Study the drawing (mm; zero at the part's minimum x, y, z) and answer. Round coordinates to 2 decimals unless told otherwise and drop trailing zeros. Write each loop counter-clockwise with the first axis right and the second up, starting at its lowest first coordinate (ties: lowest second). Pieces come first, ordered by that corner, then holes.
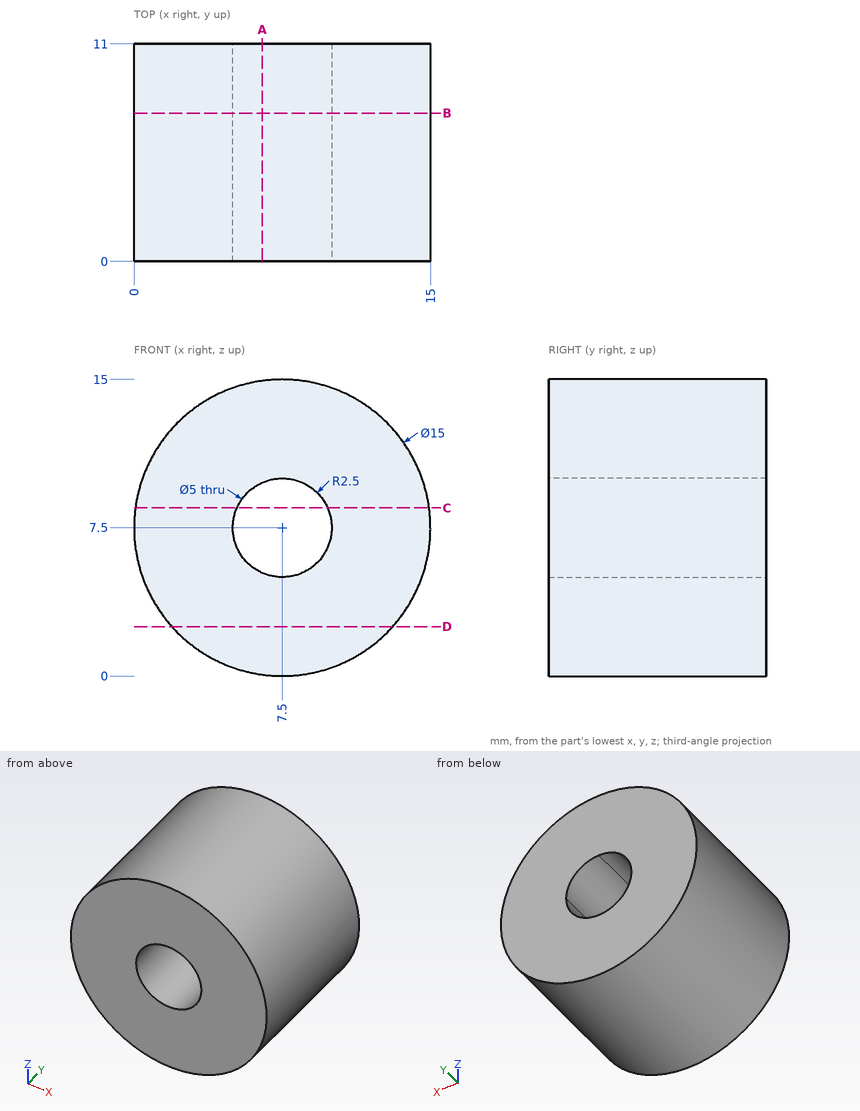
1. Straight lines are drawn through the part: line 1 along X through (y, z) = (5, 6); line 2 along Z through (x, y) = (6.25, 6.5); line 3 along Z through (x, y) = (8, 8.5). For each, find the intervals that lie inside material, in ascending order.
Geometry says:
line 1: x = 0.15 to 5.5, 9.5 to 14.85
line 2: z = 0.1 to 5.33, 9.67 to 14.9
line 3: z = 0.02 to 5.05, 9.95 to 14.98
2. Section A-A on x = 6.5 is taken. Determine the outline of the cut face in (y, z).
Geometry says:
outline: (0, 0.07) - (11, 0.07) - (11, 5.21) - (0, 5.21) - close; (0, 9.79) - (11, 9.79) - (11, 14.93) - (0, 14.93) - close
3. Given pin 1 (3 mm diameter, centred on y = 1.5, z = 13.5, fed in from -X), flat-ended and moving along its own axis, determine where the tip first touches the part or whether it passes through.
Geometry says:
pin 1: stops at x = 1.5
4. Section D-D on z = 2.5 is taken. Determine the outline of the cut face in (x, y).
Geometry says:
outline: (1.91, 0) - (13.09, 0) - (13.09, 11) - (1.91, 11) - close
5. Section C-C on z = 8.5 is taken. Determine the outline of the cut face in (x, y), plus the area to 3 significant figures.
Geometry says:
outline: (0.07, 0) - (5.21, 0) - (5.21, 11) - (0.07, 11) - close; (9.79, 0) - (14.93, 0) - (14.93, 11) - (9.79, 11) - close
area: 113 mm2
6. Section B-B on y = 7.5 is taken. Determine the outline of the cut face in (x, z), plus the area to 3 significant figures.
Geometry says:
outline: circle Ø15 at (7.5, 7.5); hole circle Ø5 at (7.5, 7.5)
area: 157 mm2
